```python
from build123d import *

# Parameters (mm, degrees)
BOSS_EXTRUDE1_DEPTH = 2
SKETCH2_R           = 1
CUT_EXTRUDE1_DEPTH  = 3.0000001


with BuildPart() as part:
    # Sketch1 → Boss-Extrude1 (new body)
    with BuildSketch(Plane(origin=(0, 0, 0), x_dir=(1, 0, 0), z_dir=(0, 1, 0))):
        with BuildLine():
            Line((5.248759298, 0.27487593), (12.5, 1))
            add(Edge.make_bspline(
                [(12.5, 1), (25.716292058, 6.056775104), (39.5099436, 6.545604881), (53.220608515, 2.413649078)],
                knots=[0, 0, 0, 0, 0.858701094, 0.858701094, 0.858701094, 0.858701094], degree=3))
            ThreePointArc((53.220608515, 2.413649078), (55.952811517, 3.321860873), (56.017920205, 6.200322748))
            add(Edge.make_bspline(
                [(16.11119686, 48.85407535), (22.252071457, 44.112915248), (36.940561271, 31.197181318), (49.405904782, 16.053895714), (56.017920205, 6.200322748)],
                knots=[0.227142679, 0.227142679, 0.227142679, 0.227142679, 0.499193547, 0.914214996, 0.914214996, 0.914214996, 0.914214996], degree=3))
            ThreePointArc((16.11119686, 48.85407535), (5.590463097, 49.913991867), (0, 40.938693304))
            add(Edge.make_bspline(
                [(0, 40.938693304), (3.065585296, 35.767628216), (2.5, 30)],
                knots=[0, 0, 0, 1, 1, 1], degree=2))
            Line((2.5, 30), (2.5, 2.762468905))
            ThreePointArc((2.5, 2.762468905), (3.322486698, 0.908837571), (5.248759298, 0.27487593))
        make_face()
    extrude(amount=BOSS_EXTRUDE1_DEPTH)

    # Sketch2 → Cut-Extrude1 (cut, through all)
    with BuildSketch(Plane(origin=(0, 2, 0), x_dir=(1, 0, 0), z_dir=(0, 1, 0))):
        with Locations((53.941981842, 4.807311653)):
            Circle(SKETCH2_R)
        with Locations((8.5, 22.807311653)):
            Circle(SKETCH2_R)
        with BuildLine():
            Line((12.575662954, 34.90249481), (12.575662954, 13.24232221))
            ThreePointArc((12.575662954, 13.24232221), (14.214859141, 10.01329676), (17.788965632, 9.430774412))
            add(Edge.make_bspline(
                [(40.437472292, 11.085030457), (37.44717133, 11.574532132), (29.837808842, 12.110288208), (22.250510571, 10.850986019), (17.788965632, 9.430774412)],
                knots=[0.180465319, 0.180465319, 0.180465319, 0.180465319, 0.4409169, 0.841911756, 0.841911756, 0.841911756, 0.841911756], degree=3))
            ThreePointArc((40.437472292, 11.085030457), (42.977221324, 12.252961632), (42.846470999, 15.045324919))
            add(Edge.make_bspline(
                [(20.840843033, 38.689129074), (25.058258326, 35.052490455), (32.827221728, 27.546668383), (39.711612857, 19.255139389), (42.846470999, 15.045324919)],
                knots=[0.21322067, 0.21322067, 0.21322067, 0.21322067, 0.550339586, 0.867457281, 0.867457281, 0.867457281, 0.867457281], degree=3))
            ThreePointArc((20.840843033, 38.689129074), (15.493104479, 39.448146601), (12.575662954, 34.90249481))
        make_face()
    extrude(amount=-CUT_EXTRUDE1_DEPTH, mode=Mode.SUBTRACT)


solid = part.part
```
Design review of the part built by this model. Coordinates are the model's own, in mm. A direction names the side the tool comes from. Coordinates: 2 decimals unless noted, no trailing zeros. Order: outer loops, then holes, each group sorted by start corner. A loop starts at its lowest first (then second) coordinate and runs counter-clockwise, first axis right, second up. Notation, with made-up numbers: M -38.5,48 L -10.5,48 A31 cw -10.5,74 Z; hole C 38.5,77.5 d5. An arc over 180 degrees is marked long. Answer as a JSON object with one key per item and string values. Group by question number.
1) Add section B-B, the plane y = 1.3. Count the separate pieces of the cut face and the enclosed holes in it, then the cut area to 3 significant figures.
2) Add section A-A, the plane x = 8.5. Write out the cut boundary in (y, z).
3) Wall thickness on L1, parallel to X at y = 1.2, z = -37.5; L2, parallel to Z at x = 23.5, y = 0.85; L3, parallel to Z at x = 41.5, y = 1.9: over which ranges is each line inside the solid? List them lowest first.
4) For pin 1 (0.6 mm diameter, centred on y = 1.5, z = -14.5, fed in from -X); pin 2 (1 mm diameter, centred on x = 31.5, y = 1, fed in from +Z); pin 3 (12 mm diameter, centred on x = 24, z = -26.5, fed in from -Y), all flat-tipped, find the tip position at first contact; note any pin that passes through.
5) Mouldability with a two-part tool opening along X and no side actions: class faces 1 (the flat face through (2.5, 1, -17)), 2 (the cylindrical face through (7.706, 1.014, -22.199)), 3 (the cylindrical face through (5.73, 0.99, -49.98)), 4 (the cylindrical face through (14.173, 1.014, -10.045)) as pulls with the +X half, pulls with the -X half, needs draft (parallel to the pull), parting line crosses it, or undercut.
6) Tool access review of faces 5 (the flat face through (9, 0, -20)), 6 (the cylindrical face through (15.566, 1.014, -39.481)): name each direction out of +Z, -Z, +X, -X, +Y, -Y from which nothing blocks a thin tool from reaching the whole face with its end or side.
Computed values:
{
 "1": {"separate pieces": "1", "enclosed holes": "3", "area": "1,100 mm^2"},
 "2": {"outline": "M 0,-50.83 L 2,-50.83 L 2,-23.81 L 0,-23.81 Z; M 0,-21.81 L 2,-21.81 L 2,-0.6 L 0,-0.6 Z"},
 "3": {"L1": "x = 1.61 to 13.3, 22.2 to 29.44", "L2": "z = -42.84 to -36.34, -10.88 to -4.13", "L3": "z = -25.05 to -16.83, -11.14 to -4.82"},
 "4": {"pin 1": "stops at x = 2.5", "pin 2": "stops at z = -5.07", "pin 3": "passes through"},
 "5": {"face 1": "pulls with the -X half", "face 2": "undercut", "face 3": "parting line crosses it", "face 4": "undercut"},
 "6": {"face 5": "+Z, -Z, +X, -X, -Y", "face 6": "+Y, -Y"}
}
